Source: CAD feature listing. Evaluate the final solid. Frame: model axes, mm. A direction names the side the tool comes from. Give positions to 0.01 mm unless a question says otherwise; leave off trailing zeros. Loops run counter-clockwise (first coordinate to the right, second up) from the corner with the lowest first, then second, coordinate; pieces in that order, holes last. Notation, with made-up numbers: (-11.5, -19) - (24.5, -19) arc R31 cw to (24.5, 18) - close; hole circle Ø5 at (53, 11.5). An arc over 180 degrees is marked (long way). Write each question's results on one line, items separated by ' | '. Start each with the question number.
(1) Material intervals for line 1 along X through (y, z) = (-15.5, -14.5); line 2 along Y through (x, z) = (24.5, -5); line 3 along Y through (x, z) = (41, -9), sorted ascending. Write a range as [from, to].
(2) Contact query for flat-ended pins moving along their axis: pin 1 (6 mm diameter, centred on x = -40.5, z = -12, fed in from +Y); pin 2 (3 mm diameter, centred on y = -17.5, z = -13.5, fed in from +X); pin 3 (12 mm diameter, centred on y = -16.5, z = -2.5, fed in from -X); pin 4 (8 mm diameter, centred on x = -35, y = -18, fed in from +Z). Output: stop coordinate, or through.
(3) Cut plane A-A on y = -23.5. Return the cut outline in (x, z), then the cut area to 3 significant figures.
(4) Reachability of faces 4 (the flat face through (-36, -13, 0)), 5 (the flat face through (36.737, -13, 0)), 6 (the flat face through (-44, -25.737, 0)) from +Z, -Z, +X, -X, +Y, -Y: full face, straight path, thin tool, end or side. Return the list, or none.
(5) Cut plane B-B on z = -5. Return the cut outline in (x, y).
(6) Cut plane C-C on x = -0.5. Return the cut outline in (y, z).
(7) Pull-direction query (X, two-part tool) for faces 1 (the flat face through (-36.737, -13, 0)), 2 (the flat face through (44, -25.737, 0)), 3 (the flat face through (36, -13, 0)); classes: pulls with the +X half, pulls with the -X half, needs draft (parallel to the pull), parting line crosses it, or undercut.
from build123d import *

# Parameters (mm, degrees)
SKETCH1_W                      = 72
SKETCH1_H                      = 35
BASE_FLANGE1_DEPTH             = 0.7366
EDGE_FLANGE1_STRIP_W           = 4.4196
EDGE_FLANGE1_STRIP_H           = 0.7366
EDGE_FLANGE1_STRIP_CUT_DEPTH   = 35
EDGE_FLANGE1_STRIP_2_W         = 4.4196
EDGE_FLANGE1_STRIP_2_H         = 0.7366
EDGE_FLANGE1_STRIP_CUT_2_DEPTH = 35
EDGE_FLANGE1_DEPTH             = 35
EDGE_FLANGE1_BEND_DEPTH        = 35
EDGE_FLANGE2_STRIP_W           = 4.4196
EDGE_FLANGE2_STRIP_H           = 0.7366
EDGE_FLANGE2_STRIP_CUT_DEPTH   = 35
EDGE_FLANGE2_STRIP_2_W         = 4.4196
EDGE_FLANGE2_STRIP_2_H         = 0.7366
EDGE_FLANGE2_STRIP_CUT_2_DEPTH = 35
EDGE_FLANGE2_DEPTH             = 35
EDGE_FLANGE2_BEND_DEPTH        = 35


# Sheet-metal steps are written as plain solids
with BuildPart() as part:
    # Sketch1 → Base-Flange1 (new body)
    with BuildSketch(Plane(origin=(0, 0, 0), x_dir=(1, 0, 0), z_dir=(0, 1, 0))):
        Rectangle(SKETCH1_W, SKETCH1_H)
    extrude(amount=-BASE_FLANGE1_DEPTH)

    # Edge-Flange1 strip (across the edge) → Edge-Flange1 strip cut (cut)
    with BuildSketch(Plane(origin=(36, -0.7366, -17.5), x_dir=(-1, 0, 0), z_dir=(0, 0, 1))):
        with Locations((-1.4732, -0.3683)):
            Rectangle(EDGE_FLANGE1_STRIP_W, EDGE_FLANGE1_STRIP_H)
    extrude(amount=EDGE_FLANGE1_STRIP_CUT_DEPTH, mode=Mode.SUBTRACT)

    # Edge-Flange1 strip 2 (across the edge) → Edge-Flange1 strip cut 2 (cut)
    with BuildSketch(Plane(origin=(-36, -0.7366, 17.5), x_dir=(1, 0, 0), z_dir=(0, 0, -1))):
        with Locations((-1.4732, -0.3683)):
            Rectangle(EDGE_FLANGE1_STRIP_2_W, EDGE_FLANGE1_STRIP_2_H)
    extrude(amount=EDGE_FLANGE1_STRIP_CUT_2_DEPTH, mode=Mode.SUBTRACT)

    # Edge-Flange1 section (across the edge) → Edge-Flange1 (add)
    with BuildSketch(Plane(origin=(36, -0.7366, -17.5), x_dir=(-1, 0, 0), z_dir=(0, 0, 1))):
        with BuildLine():
            Line((-0.7366, 0.7366), (-0.7366, 25))
            Line((-0.7366, 25), (0, 25))
            Line((0, 25), (0, 0.7366))
            ThreePointArc((0, 0.7366), (0.215745145, 0.215745145), (0.7366, 0))
            Line((0.7366, 0), (0.7366, -0.7366))
            ThreePointArc((0.7366, -0.7366), (-0.30510971, -0.30510971), (-0.7366, 0.7366))
        make_face()
    extrude(amount=EDGE_FLANGE1_DEPTH)

    # Edge-Flange1 section 2 (across the edge) → Edge-Flange1 bend (add)
    with BuildSketch(Plane(origin=(-36, -0.7366, 17.5), x_dir=(1, 0, 0), z_dir=(0, 0, -1))):
        with BuildLine():
            Line((-0.7366, 0.7366), (-0.7366, 25))
            Line((-0.7366, 25), (0, 25))
            Line((0, 25), (0, 0.7366))
            ThreePointArc((0, 0.7366), (0.215745145, 0.215745145), (0.7366, 0))
            Line((0.7366, 0), (0.7366, -0.7366))
            ThreePointArc((0.7366, -0.7366), (-0.30510971, -0.30510971), (-0.7366, 0.7366))
        make_face()
    extrude(amount=EDGE_FLANGE1_BEND_DEPTH)

    # Edge-Flange2 strip (across the edge) → Edge-Flange2 strip cut (cut)
    with BuildSketch(Plane(origin=(-36.7366, -25.7366, -17.5), x_dir=(0, 1, 0), z_dir=(0, 0, 1))):
        with Locations((-1.4732, -0.3683)):
            Rectangle(EDGE_FLANGE2_STRIP_W, EDGE_FLANGE2_STRIP_H)
    extrude(amount=EDGE_FLANGE2_STRIP_CUT_DEPTH, mode=Mode.SUBTRACT)

    # Edge-Flange2 strip 2 (across the edge) → Edge-Flange2 strip cut 2 (cut)
    with BuildSketch(Plane(origin=(36.7366, -25.7366, 17.5), x_dir=(0, 1, 0), z_dir=(0, 0, -1))):
        with Locations((-1.4732, -0.3683)):
            Rectangle(EDGE_FLANGE2_STRIP_2_W, EDGE_FLANGE2_STRIP_2_H)
    extrude(amount=EDGE_FLANGE2_STRIP_CUT_2_DEPTH, mode=Mode.SUBTRACT)

    # Edge-Flange2 section (across the edge) → Edge-Flange2 (add)
    with BuildSketch(Plane(origin=(-36.7366, -25.7366, -17.5), x_dir=(0, 1, 0), z_dir=(0, 0, 1))):
        with BuildLine():
            Line((-0.7366, 0.7366), (-0.7366, 14.2634))
            Line((-0.7366, 14.2634), (0, 14.2634))
            Line((0, 14.2634), (0, 0.7366))
            ThreePointArc((0, 0.7366), (0.215745145, 0.215745145), (0.7366, 0))
            Line((0.7366, 0), (0.7366, -0.7366))
            ThreePointArc((0.7366, -0.7366), (-0.30510971, -0.30510971), (-0.7366, 0.7366))
        make_face()
    extrude(amount=EDGE_FLANGE2_DEPTH)

    # Edge-Flange2 section 2 (across the edge) → Edge-Flange2 bend (add)
    with BuildSketch(Plane(origin=(36.7366, -25.7366, 17.5), x_dir=(0, 1, 0), z_dir=(0, 0, -1))):
        with BuildLine():
            Line((-0.7366, 0.7366), (-0.7366, 14.2634))
            Line((-0.7366, 14.2634), (0, 14.2634))
            Line((0, 14.2634), (0, 0.7366))
            ThreePointArc((0, 0.7366), (0.215745145, 0.215745145), (0.7366, 0))
            Line((0.7366, 0), (0.7366, -0.7366))
            ThreePointArc((0.7366, -0.7366), (-0.30510971, -0.30510971), (-0.7366, 0.7366))
        make_face()
    extrude(amount=EDGE_FLANGE2_BEND_DEPTH)


solid = part.part
Ans:
1) line 1: [-36.74, -36], [36, 36.74] | line 2: [-0.74, 0] | line 3: [-26.47, -25.74]
2) pin 1: y = -25.74 | pin 2: x = 36.74 | pin 3: x = -36.74 | pin 4: z = 17.5
3) outline: (-36.74, -17.5) - (-36, -17.5) - (-36, 17.5) - (-36.74, 17.5) - close; (36, -17.5) - (36.74, -17.5) - (36.74, 17.5) - (36, 17.5) - close | area: 51.6 mm^2
4) face 4: +Z, -Z, -Y | face 5: +Z, -Z, +X, +Y | face 6: +Z, -Z, -X, +Y
5) outline: (-51, -26.47) - (-37.47, -26.47) arc R1.47 ccw to (-36, -25) - (-36, -1.47) arc R0.74 cw to (-35.26, -0.74) - (35.26, -0.74) arc R0.74 cw to (36, -1.47) - (36, -25) arc R1.47 ccw to (37.47, -26.47) - (51, -26.47) - (51, -25.74) - (37.47, -25.74) arc R0.74 cw to (36.74, -25) - (36.74, -1.47) arc R1.47 ccw to (35.26, 0) - (-35.26, 0) arc R1.47 ccw to (-36.74, -1.47) - (-36.74, -25) arc R0.74 cw to (-37.47, -25.74) - (-51, -25.74) - close
6) outline: (-0.74, -17.5) - (0, -17.5) - (0, 17.5) - (-0.74, 17.5) - close
7) face 1: pulls with the -X half | face 2: needs draft | face 3: undercut
